Input: part model. Units: mm. Frame: model coordinates. A direction names the side the tool comes from. Give positions to 0.01 mm unless a question says otherwise; leave off trailing zeros. Loops run counter-clockwise (first coordinate to the right, second up) from the corner with the lowest first, then second, coordinate; pieces in that order, holes last.
Autodesk Inventor part; units mm, degrees
ref_plane "YZ Plane" through (0, 0, 0) normal (1, 0, 0) x (0, 1, 0)
ref_plane "XZ Plane" through (0, 0, 0) normal (0, 1, 0) x (-1, 0, 0)
ref_plane "XY Plane" through (0, 0, 0) normal (0, 0, 1) x (1, 0, 0)
sketch "Sketch1" plane through (0, 0, 0) normal (0, 0, 1) x (1, 0, 0)
  arc A0 (0.1634, -106.6592) -> (254.828, -79.7002) centre (0.1634, 1109.6463) ccw
  arc A1 (0.1634, -121.6592) -> (244.7719, -97.118) centre (0.1634, 1109.6463) ccw
  line L0 (254.828, -79.7002) -> (244.7719, -97.118)
  line L1 (254.828, -79.7002) -> (274.9404, -79.7002) construction
  line L2 (0.1634, -121.6592) -> (0.1634, -88.4091)
  arc A2 (-244.445, -97.118) -> (0.1634, -121.6592) centre (0.1634, 1109.6463) ccw
  arc A3 (-254.5012, -79.7002) -> (0.1634, -106.6592) centre (0.1634, 1109.6463) ccw
  line L3 (-254.5012, -79.7002) -> (-244.445, -97.118)
  point P0 (0, 0)
  point P1 (226.5563, -100.6675)
  dimension "d0" = 15
  dimension "d1" = 120
extrude "Extrusion1" add sketch "Sketch1" along normal blind 30
fillet "Fillet1" radius 3 12 edges at (-127.8803, -99.9007, 30) (123.0817, -115.5086, 30) (128.2072, -99.9007, 0) (249.8, -88.4091, 30) (254.828, -79.7002, 15) (244.7719, -97.118, 15) (249.8, -88.4091, 0) (123.0817, -115.5086, 0) (-249.4731, -88.4091, 0) (-244.445, -97.118, 15) (-249.4731, -88.4091, 30) (-254.5012, -79.7002, 15)
sketch "Sketch2" plane through (0, 0, 0) normal (0, 1, 0) x (-1, 0, 0)
  line L0 (0, 0) -> (0, 15)
  circle A0 centre (0, 15) radius 5
  dimension "d5" = 15
  dimension "d6" = 10
extrude "Extrusion2" cut sketch "Sketch2" against normal blind 300
properties part number "leaf 4" material "Steel, Carbon"
(1) Ray query, probe 1 along Z at (x, y) = (0, -117.75); probe 2 along Y at (x, z) = (7.5, 16.5); probe 3 along Y at (x, z) = (148.5, 26). Return the intervals inside material, ascending.
Values follow:
probe 1: z = 0 to 10, 20 to 30
probe 2: y = -121.64 to -106.64
probe 3: y = -112.69 to -97.58
(2) Pin query (flat end, axial travel): pin 1 Ø4 at (y, z) = (-86.5, 4.5) entering from -X; pin 2 Ø5 at (y, z) = (-98.5, 15) entering from -X. Return the tip coordinate at first contact, or that it passes through.
Values follow:
pin 1: stops at x = -251.5
pin 2: stops at x = -245.09
(3) Cut plane A-A (z = 15). Return the cut outline in (x, y).
Values follow:
outline: (-251.14, -85.53) - (-245.12, -95.95) arc R3 ccw to (-243.12, -97.39) arc R1231.3 ccw to (-5, -121.65) - (-5, -106.65) arc R1216.3 cw to (-247.93, -81.09) arc R3 ccw to start; (5, -121.65) arc R1231.31 ccw to (243.44, -97.39) arc R3 ccw to (245.45, -95.95) - (251.46, -85.53) arc R3 ccw to (248.25, -81.09) arc R1216.31 cw to (5, -106.65) - close
(4) Mould query, pull axis X, two halves, no side actions, for faces 1 (the flat face through (-1, -110, 30)), 2 (the cylindrical face through (248, -90, 29)), 3 (the cylindrical face through (-122.8, -100.428, 14.832)), 4 (the cylindrical face through (1.08, -114.05, 10.12)). Classes: +X half, -X half, draft (parallel to the pull), parting line (faces both ways), or undercut.
Values follow:
face 1: draft
face 2: +X half
face 3: undercut
face 4: undercut
(5) Reachability of faces 5 (the cylindrical face through (124.113, -115.405, 14.832)), 6 (the cylindrical face through (126.61, -100.07, 14.83)) from +Z, -Z, +X, -X, +Y, -Y: full face, straight path, thin tool, end or side. Return the list, or none.
Values follow:
face 5: +Z, -Z, +X, -Y
face 6: +Z, -Z, +Y
